Design review of the part built by this model. Coordinates are the model's own, in mm. A direction names the side the tool comes from. Round coordinates to 2 decimals unless told otherwise and drop trailing zeros. Loops run counter-clockwise (first coordinate to the right, second up) from the corner with the lowest first, then second, coordinate; pieces in that order, holes last. Notation, with made-up numbers: (37, 65) -> (79, 65) arc R20 ccw to (79, 82) -> close; hole circle Ø1 at (19.25, -0.75). An arc over 180 degrees is marked (long way). Use a Markdown table: item, result. Add a question column.
from build123d import *

# Parameters (mm, degrees)
SKETCH1_R               = 16.66875
BOSS_EXTRUDE1_DEPTH     = 69.85
CUT_EXTRUDE1_DEPTH      = 74.720532778
CUT_EXTRUDE1_DEPTH_BACK = 26.9875
SKETCH3_R               = 13.49375
SKETCH4_R               = 16.66875
BOSS_EXTRUDE2_DEPTH     = 34.925
SKETCH5_R               = 12.7
CUT_EXTRUDE2_DEPTH      = 101.179300459
CUT_EXTRUDE8_START      = 19.05
SKETCH11_R              = 13.49375
CUT_EXTRUDE8_DEPTH      = 19.05
CUT_EXTRUDE5_DEPTH      = 80.853774811
CUT_EXTRUDE5_DEPTH_BACK = 80.853774811
SKETCH10_R              = 12.7
SKETCH13_R              = 13.49375
CUT_EXTRUDE9_DEPTH      = 19.05
CUT_EXTRUDE10_START     = -19.05
SKETCH14_R              = 13.49375
CUT_EXTRUDE10_DEPTH     = 19.05
SKETCH15_R              = 16.66875
BOSS_EXTRUDE3_DEPTH     = 34.925
SKETCH17_R              = 13.49375
CUT_EXTRUDE12_DEPTH     = 19.05
SKETCH19_R              = 12.7
CUT_EXTRUDE14_DEPTH     = 105.775000133
SKETCH20_R              = 12.7
CUT_EXTRUDE15_DEPTH     = 86.548429389
SKETCH22_R              = 12.7
CUT_EXTRUDE16_DEPTH     = 30.48


with BuildPart() as part:
    # Sketch1 → Boss-Extrude1 (new body)
    with BuildSketch(Plane.XY):
        Circle(SKETCH1_R)
    extrude(amount=BOSS_EXTRUDE1_DEPTH)

    # Sketch3 → Cut-Extrude1 (cut, two sides: drawn at the far end of the back side and taken through both)
    with BuildSketch(Plane.XY.offset(69.85).offset(-CUT_EXTRUDE1_DEPTH_BACK)):
        with Locations(Location((0, 0, 0), (0, 0, 180))):
            Circle(SKETCH3_R)
    extrude(amount=CUT_EXTRUDE1_DEPTH + CUT_EXTRUDE1_DEPTH_BACK, mode=Mode.SUBTRACT)

    # Sketch4 → Boss-Extrude2 (add, symmetric)
    with BuildSketch(Plane(origin=(0, 0, 0), x_dir=(0, 0, -1), z_dir=(1, 0, 0))):
        with Locations(Location((-34.925, 0, 0), (0, 0, 270))):
            Circle(SKETCH4_R)
    extrude(amount=BOSS_EXTRUDE2_DEPTH, both=True)

    # Sketch5 → Cut-Extrude2 (cut, through all)
    with BuildSketch(Plane(origin=(34.925, 0, 0), x_dir=(0, 0, -1), z_dir=(1, 0, 0))):
        with Locations((-34.925, 0)):
            Circle(SKETCH5_R)
    extrude(amount=-CUT_EXTRUDE2_DEPTH, mode=Mode.SUBTRACT)

    # Sketch11 → Cut-Extrude8 (cut)
    with BuildSketch(Plane.XY.offset(CUT_EXTRUDE8_START)):
        with Locations(Location((0, 0, 0), (0, 0, 180))):
            Circle(SKETCH11_R)
    extrude(amount=-CUT_EXTRUDE8_DEPTH, mode=Mode.SUBTRACT)

    # Sketch10 → Cut-Extrude5 (cut, two sides: drawn at the far end of the back side and taken through both)
    with BuildSketch(Plane.XY.offset(69.85).offset(-CUT_EXTRUDE5_DEPTH_BACK)):
        Circle(SKETCH10_R)
    extrude(amount=CUT_EXTRUDE5_DEPTH + CUT_EXTRUDE5_DEPTH_BACK, mode=Mode.SUBTRACT)

    # Sketch13 → Cut-Extrude9 (cut)
    with BuildSketch(Plane(origin=(34.925, 0, 0), x_dir=(0, 0, -1), z_dir=(1, 0, 0))):
        with Locations((-34.925, 0)):
            Circle(SKETCH13_R)
    extrude(amount=-CUT_EXTRUDE9_DEPTH, mode=Mode.SUBTRACT)

    # Sketch14 → Cut-Extrude10 (cut)
    with BuildSketch(Plane.ZY.offset(34.925).offset(CUT_EXTRUDE10_START)):
        with Locations(Location((34.925, 0, 0), (0, 0, 180))):
            Circle(SKETCH14_R)
    extrude(amount=CUT_EXTRUDE10_DEPTH, mode=Mode.SUBTRACT)

    # Sketch15 → Boss-Extrude3 (add)
    with BuildSketch(Plane(origin=(0, 0, 0), x_dir=(1, 0, 0), z_dir=(0, 1, 0))):
        with Locations(Location((0, -34.925, 0), (0, 0, 107.752790162))):
            Circle(SKETCH15_R)
    extrude(amount=BOSS_EXTRUDE3_DEPTH)

    # Sketch17 → Cut-Extrude12 (cut)
    with BuildSketch(Plane(origin=(0, 34.925, 0), x_dir=(1, 0, 0), z_dir=(0, 1, 0))):
        with Locations(Location((0, -34.925, 0), (0, 0, 270))):
            Circle(SKETCH17_R)
    extrude(amount=-CUT_EXTRUDE12_DEPTH, mode=Mode.SUBTRACT)

    # Sketch19 → Cut-Extrude14 (cut, through all)
    with BuildSketch(Plane(origin=(34.925, 0, 0), x_dir=(0, 0, -1), z_dir=(1, 0, 0))):
        with Locations(Location((-34.925, 0, 0), (0, 0, 66.409614008))):
            Circle(SKETCH19_R)
    extrude(amount=-CUT_EXTRUDE14_DEPTH, mode=Mode.SUBTRACT)

    # Sketch20 → Cut-Extrude15 (cut, through all)
    with BuildSketch(Plane.XY.offset(69.85)):
        with Locations(Location((0, 0, 0), (0, 0, 113.590385992))):
            Circle(SKETCH20_R)
    extrude(amount=-CUT_EXTRUDE15_DEPTH, mode=Mode.SUBTRACT)

    # Sketch22 → Cut-Extrude16 (cut)
    with BuildSketch(Plane(origin=(0, 34.925, 0), x_dir=(1, 0, 0), z_dir=(0, 1, 0))):
        with Locations(Location((0, -34.925, 0), (0, 0, 270))):
            Circle(SKETCH22_R)
    extrude(amount=-CUT_EXTRUDE16_DEPTH, mode=Mode.SUBTRACT)


solid = part.part
1. For faces 4 (the face through (15.875, -13, 35)), 5 (the face through (-3.613, -16.272, 9.457)), 6 (the face through (0.558, 13.242, 22.237)), list the 3-axis set-ups (+Z, -Z, +X, -X, +Y, -Y) from which the entire face can be reached by the end or side of a thin tool; tool diameter is ignored.
2. To check wall thickness, follow probe 1 along Z at (x, y) = (23, 0); probe 2 along X at (y, z) = (12, 7); probe 3 along Y at (x, z) = (0, 39). State the ranges of each line that lie inside material, in increasing order. Write a range as from..to.
3. Consider section B-B on y = 0. Give the number of separate pieces and of enclosed holes in the cut face, plus the area to 3 significant figures.
4. Consider section D-D on x = 18.5. State the section outline as (y, z) points (1 decimal), plus the area to 3 significant figures.
5. Mouldability with a two-part tool opening along Y and no side actions: class faces 1 (the face through (-24.98, -15.9, 29.92)), 2 (the face through (3.063, -12.561, 45.883)), 3 (the face through (-8, 15.875, 45)) as +Y half, -Y half, draft (parallel to the pull), parting line (faces both ways), or undercut.
6. Consider section A-A on z = 57. State the section outline as (x, y) points, plus the area to 3 significant figures.
7. Insertion check: P1, Ø1.5, axis at x = -2.5, y = 18.5, coming from the -Z side; P2, Ø13.5, axis at x = 2.5, z = 37.5, coming from the +Y side; P3, Ø2, axis at x = 20.5, y = -5.5, coming from the +Z side. Each pin has a flat end and moves straight along its axis. Give the tip position at first contact, or say it passes through.
Verdict:
| question | item | result |
|---|---|---|
| 1 | face 4 | +X |
| 1 | face 5 | -Z |
| 1 | face 6 | +Y |
| 2 | probe 1 | z = 18.26..21.43, 48.42..51.59 |
| 2 | probe 2 | x = -11.57..-6.17, 6.17..11.57 |
| 2 | probe 3 | y = -16.67..-12.7 |
| 3 | separate pieces | 4 |
| 3 | enclosed holes | 0 |
| 3 | area | 523 mm² |
| 4 | outline | circle Ø33.3 at (0, 34.9); hole circle Ø27 at (0, 34.9) |
| 4 | area | 301 mm² |
| 5 | face 1 | parting line |
| 5 | face 2 | undercut |
| 5 | face 3 | +Y half |
| 6 | outline | circle Ø33.34 at (0, 0); hole circle Ø26.99 at (0, 0) |
| 6 | area | 301 mm² |
| 7 | P1 | stops at z = 18.35 |
| 7 | P2 | stops at y = -10.39 |
| 7 | P3 | stops at z = 50.97 |
